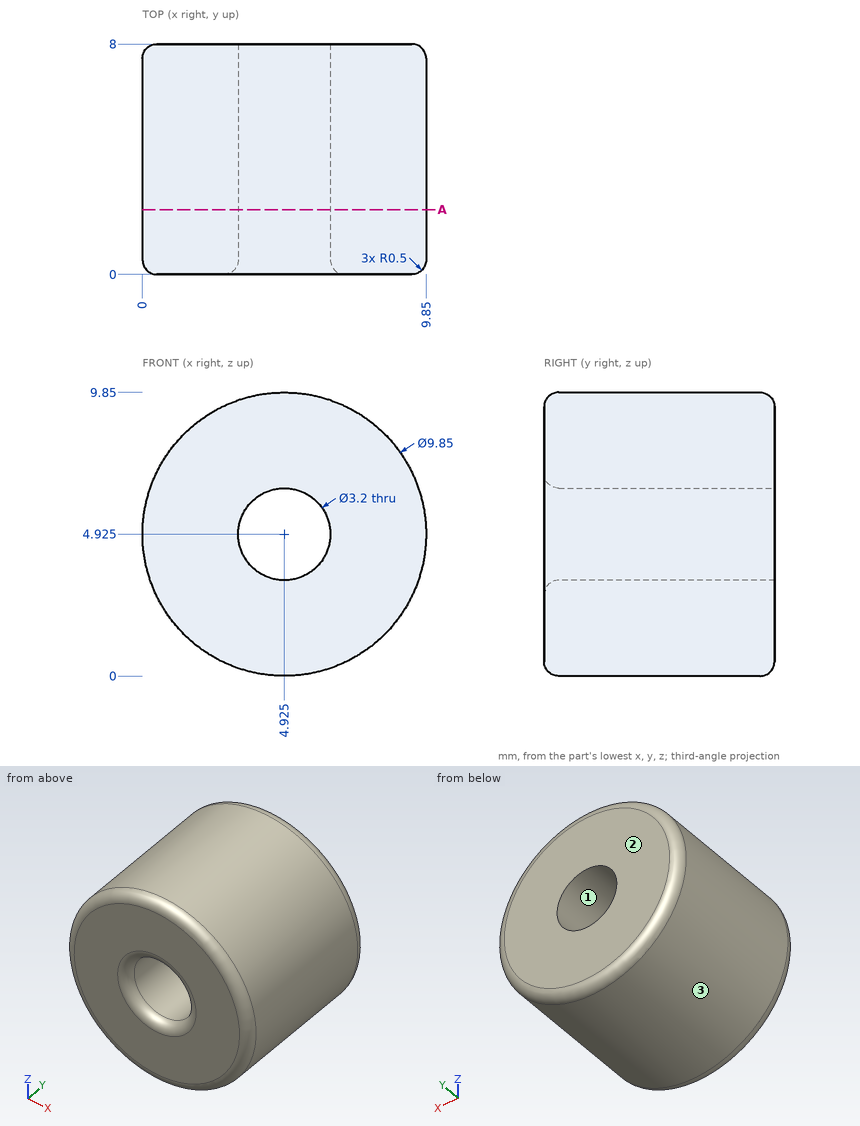
Job drawing, mm, ordinate dimensions from the low corner. One solid piece. Coordinates: 2 decimals unless noted, no trailing zeros. Order: outer loops, then holes, each group sorted by start corner. A loop starts at its lowest first (then second) coordinate and runs counter-clockwise, first axis right, second up. Notation, with made-up numbers: (3, 49) -> (15, 49) arc R28 ccw to (15, 80) -> close; hole circle Ø5 at (80, 22). An arc over 180 degrees is marked (long way). Put each result on its own line as item: value. Start each with the question number.
(1) Band-saw the part on A-A (y = 2.25). Give the cut face in (x, z) (3 decimals).
(2) Pin check, flat tips, straight feed: pin 1 Ø4 at (x, z) = (4.925, 4.925) entering from -Y; pin 2 Ø3 at (x, y) = (4.5, 4.5) entering from +Z; pin 3 Ø4 at (y, z) = (2, 8) entering from +X; pin 4 Ø3 at (y, z) = (3.5, 8) entering from +X. Stop position of each tip, or through.
(3) Probe line 1 along Z through (x, y) = (5, 4.5); line 2 along X through (y, z) = (5, 3.5); line 3 along Z through (x, y) = (4.5, 1.25). List the from-to ranges inside material, lowest first. Write a range as [from, to].
(4) Mould opens along X. For the marked faces 1, 2 and 3 say: pulls with the +X half, pulls with the -X half, needs draft (parallel to the pull), parting line crosses it, or undercut.
Determined:
1. outline: circle Ø9.85 at (4.925, 4.925); hole circle Ø3.2 at (4.925, 4.925)
2. pin 1: stops at y = 0.01
2. pin 2: stops at z = 9.85
2. pin 3: stops at x = 9.73
2. pin 4: stops at x = 9.59
3. line 1: z = [0, 3.33], [6.52, 9.85]
3. line 2: x = [0.21, 4.2], [5.65, 9.64]
3. line 3: z = [0.02, 3.38], [6.47, 9.83]
4. face 1: undercut
4. face 2: needs draft
4. face 3: parting line crosses it
